Here's how the part is built. I have some questions about the finished solid (model axes, mm). Coordinates: 2 decimals unless noted, no trailing zeros.
```python
from build123d import *

# Parameters (mm, degrees)
SKETCH_1_W                   = 680
SKETCH_1_H                   = 24
EXTRUDE_1_DEPTH              = 8.5
HOLE_WIZARD_M4_1_D           = 4.8
HOLE_WIZARD_M4_1_CBORE_D     = 8
HOLE_WIZARD_M4_1_CBORE_DEPTH = 4
PATTERN_LINEAR_1_COUNT       = 17
PATTERN_LINEAR_1_PITCH       = 40


with BuildPart() as part:
    # 草图1 → 凸台-拉伸1 (new body)
    with BuildSketch(Plane.XY):
        with Locations((340, 12)):
            Rectangle(SKETCH_1_W, SKETCH_1_H)
    extrude(amount=EXTRUDE_1_DEPTH)

    # M4 六角凹头螺钉的柱形沉头孔1 (through all)
    with Locations(Plane.XY.offset(8.5)):
        with Locations((20, 12)):
            hole_wizard_m4_1 = CounterBoreHole(HOLE_WIZARD_M4_1_D / 2, HOLE_WIZARD_M4_1_CBORE_D / 2, HOLE_WIZARD_M4_1_CBORE_DEPTH)

    # 阵列(线性)1: M4 六角凹头螺钉的柱形沉头孔1 ×17
    with Locations(*[(i * PATTERN_LINEAR_1_PITCH, 0, 0) for i in range(1, PATTERN_LINEAR_1_COUNT)]):
        add(hole_wizard_m4_1, mode=Mode.SUBTRACT)


solid = part.part
```
1) I need wall thicknesses on probe 1 along Y at (x, z) = (620, 7.5); probe 2 along Y at (x, z) = (580, 1.75); probe 3 along Z at (x, y) = (377, 11.5). Which ranges of each line are inside material? Lowest first, please.
Values follow:
probe 1: y = 0 to 8, 16 to 24
probe 2: y = 0 to 9.6, 14.4 to 24
probe 3: z = 0 to 4.5
2) Imagine slicing it at A-A on z = 3. Count the separate pieces of the cut face and the enclosed holes in it, then the cut area to 3 significant figures.
Values follow:
separate pieces: 1
enclosed holes: 17
area: 16,000 mm2
3) Will this pin go through, and if not, where does the flat tip stop? pin 1 (2.5 mm diameter, centred on x = 179.5, y = 10.5, fed in from +Z).
Values follow:
pin 1: stops at z = 4.5
